Build history of the part. All positions in model axes, mm. Coordinates: 2 decimals unless noted, no trailing zeros. Write each loop counter-clockwise with the first axis right and the second up, starting at its lowest first coordinate (ties: lowest second). Pieces come first, ordered by that corner, then holes.
```python
from build123d import *

# Parameters (mm, degrees)
SKETCH1_W           = 650
SKETCH1_H           = 137.5
BOSS_EXTRUDE1_DEPTH = 3
SKETCH2_R           = 43.5
CUT_EXTRUDE1_DEPTH  = 384.084433891
SKETCH2_3_R         = 43.5
SKETCH2_3_R_2       = 10
CUT_EXTRUDE2_DEPTH  = 10


with BuildPart() as part:
    # Sketch1 → Boss-Extrude1 (new body)
    with BuildSketch(Plane(origin=(0, 0, 0), x_dir=(1, 0, 0), z_dir=(0, 1, 0))):
        with Locations((28.149606299, -79.67519685)):
            Rectangle(SKETCH1_W, SKETCH1_H)
    extrude(amount=BOSS_EXTRUDE1_DEPTH)

    # Sketch2 → Cut-Extrude1 (cut, through all)
    with BuildSketch(Plane(origin=(0, 3, 0), x_dir=(1, 0, 0), z_dir=(0, 1, 0))):
        with Locations(Location((-236.850393701, -70.92519685, 0), (0, 0, 270))):
            Circle(SKETCH2_R)
        with Locations(Location((-130.850393701, -70.92519685, 0), (0, 0, 270))):
            Circle(SKETCH2_R)
        with Locations(Location((-24.850393701, -70.92519685, 0), (0, 0, 270))):
            Circle(SKETCH2_R)
        with Locations(Location((81.149606299, -70.92519685, 0), (0, 0, 270))):
            Circle(SKETCH2_R)
        with Locations(Location((187.149606299, -70.92519685, 0), (0, 0, 270))):
            Circle(SKETCH2_R)
        with Locations(Location((293.149606299, -70.92519685, 0), (0, 0, 270))):
            Circle(SKETCH2_R)
    extrude(amount=-CUT_EXTRUDE1_DEPTH, mode=Mode.SUBTRACT)

    # Sketch2_3 → Cut-Extrude2 (cut)
    with BuildSketch(Plane(origin=(0, 3, 0), x_dir=(1, 0, 0), z_dir=(0, 1, 0))):
        with Locations(Location((-236.850393701, -70.92519685, 0), (0, 0, 270))):
            Circle(SKETCH2_3_R)
        with Locations(Location((-130.850393701, -70.92519685, 0), (0, 0, 270))):
            Circle(SKETCH2_3_R)
        with Locations(Location((-24.850393701, -70.92519685, 0), (0, 0, 270))):
            Circle(SKETCH2_3_R)
        with Locations(Location((81.149606299, -70.92519685, 0), (0, 0, 270))):
            Circle(SKETCH2_3_R)
        with Locations(Location((187.149606299, -70.92519685, 0), (0, 0, 270))):
            Circle(SKETCH2_3_R)
        with Locations(Location((293.149606299, -70.92519685, 0), (0, 0, 270))):
            Circle(SKETCH2_3_R)
        with Locations((338.149606299, -20.92419685)):
            Circle(SKETCH2_3_R_2)
    extrude(amount=-CUT_EXTRUDE2_DEPTH, mode=Mode.SUBTRACT)


solid = part.part
```
1. Mould opens along Z. For faces 1 (the face through (-101.451, 1.521, 38.864)), 2 (the face through (24, 0, 79)) say: +Z half, -Z half, draft (parallel to the pull), parting line (faces both ways), or undercut.
Computed values:
face 1: undercut
face 2: draft
2. Saw through at A-A on x = 257. List the corners of the cut face in (y, z), plus the area to 3 significant figures.
Computed values:
outline: (0, 10.93) - (3, 10.93) - (3, 46.73) - (0, 46.73) - close; (0, 95.12) - (3, 95.12) - (3, 148.43) - (0, 148.43) - close
area: 267 mm2
3. Saw through at C-C on y = 2.4. List the corners of the cut face in (x, z), plus the area to 3 significant figures.
Computed values:
outline: (-296.85, 10.93) - (338.01, 10.93) arc R10 cw (long way) to (338.29, 10.93) - (353.15, 10.93) - (353.15, 148.43) - (-296.85, 148.43) - close; hole circle Ø87 at (-236.85, 70.93); hole circle Ø87 at (-130.85, 70.93); hole circle Ø87 at (-24.85, 70.93); hole circle Ø87 at (81.15, 70.93); hole circle Ø87 at (187.15, 70.93); hole circle Ø87 at (293.15, 70.93)
area: 53,400 mm2
4. Saw through at B-B on z = 79. List the corners of the cut face in (x, y), plus the area to 3 significant figures.
Computed values:
outline: (-296.85, 0) - (-279.59, 0) - (-279.59, 3) - (-296.85, 3) - close; (-194.11, 0) - (-173.59, 0) - (-173.59, 3) - (-194.11, 3) - close; (-88.11, 0) - (-67.59, 0) - (-67.59, 3) - (-88.11, 3) - close; (17.89, 0) - (38.41, 0) - (38.41, 3) - (17.89, 3) - close; (123.89, 0) - (144.41, 0) - (144.41, 3) - (123.89, 3) - close; (229.89, 0) - (250.41, 0) - (250.41, 3) - (229.89, 3) - close; (335.89, 0) - (353.15, 0) - (353.15, 3) - (335.89, 3) - close
area: 411 mm2
5. Saw through at D-D on x = 71. List the corners of the cut face in (y, z).
Computed values:
outline: (0, 10.93) - (3, 10.93) - (3, 28.63) - (0, 28.63) - close; (0, 113.22) - (3, 113.22) - (3, 148.43) - (0, 148.43) - close
6. Probe line 1 along Z through (x, y) = (-24, 2.35); line 2 along Z through (x, y) = (291, 2.8). List the from-to ranges inside material, lowest first.
Computed values:
line 1: z = 10.93 to 27.43, 114.42 to 148.43
line 2: z = 10.93 to 27.48, 114.37 to 148.43
